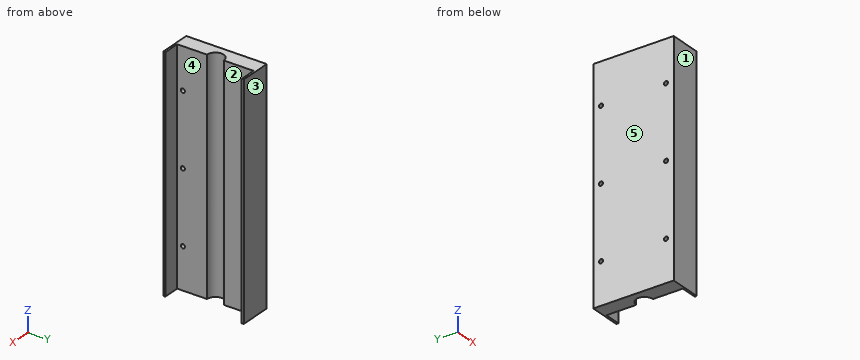
```python
from build123d import *

# Parameters (mm, degrees)
SALIENTE_EXTRUIR1_DEPTH   = 220
CROQUIS5_R                = 2
CORTAR_EXTRUIR5_DEPTH     = 20
CROQUIS7_W                = 220
CROQUIS7_H                = 2
SALIENTE_EXTRUIR2_DEPTH   = 16
SALIENTE_EXTRUIR2_2_DEPTH = 16
CROQUIS7_3_W              = 220
CROQUIS7_3_H              = 2
SALIENTE_EXTRUIR3_DEPTH   = 15


with BuildPart() as part:
    # Croquis1 → Saliente-Extruir1 (new body)
    with BuildSketch(Plane.XY):
        with BuildLine():
            Line((0, 37), (0, 8.15))
            ThreePointArc((0, 8.15), (-8.15, 0), (0, -8.15))
            Line((0, -8.15), (0, -37))
            Line((0, -37), (-15, -37))
            Line((-15, -37), (-15, 37))
            Line((-15, 37), (0, 37))
        make_face()
    extrude(amount=SALIENTE_EXTRUIR1_DEPTH)

    # Croquis5 → Cortar-Extruir5 (cut)
    with BuildSketch(Plane.ZY.offset(15)):
        with Locations((110, -31.5)):
            Circle(CROQUIS5_R)
        with Locations((110, 31.5)):
            Circle(CROQUIS5_R)
        with Locations((40, 31.5)):
            Circle(CROQUIS5_R)
        with Locations((40, -31.5)):
            Circle(CROQUIS5_R)
        with Locations((180, 31.5)):
            Circle(CROQUIS5_R)
        with Locations((180, -31.5)):
            Circle(CROQUIS5_R)
    extrude(amount=-CORTAR_EXTRUIR5_DEPTH, mode=Mode.SUBTRACT)



with BuildPart() as body_2:
    # Croquis7 → Saliente-Extruir2 (new body)
    with BuildSketch(Plane(origin=(0, 0, 0), x_dir=(0, 0, -1), z_dir=(1, 0, 0))):
        with Locations((-110, -38)):
            Rectangle(CROQUIS7_W, CROQUIS7_H)
    extrude(amount=SALIENTE_EXTRUIR2_DEPTH)


with BuildPart() as body_3:
    # Croquis7 → Saliente-Extruir2 2 (new body)
    with BuildSketch(Plane(origin=(0, 0, 0), x_dir=(0, 0, -1), z_dir=(1, 0, 0))):
        with Locations((-110, 38)):
            Rectangle(CROQUIS7_W, CROQUIS7_H)
    extrude(amount=SALIENTE_EXTRUIR2_2_DEPTH)


with BuildPart() as part_1:
    add(part.part)

    add(body_2.part)  # Saliente-Extruir3 merges body 2

    add(body_3.part)  # Saliente-Extruir3 merges body 3
    # Croquis7_3 → Saliente-Extruir3 (add)
    with BuildSketch(Plane(origin=(0, 0, 0), x_dir=(0, 0, -1), z_dir=(1, 0, 0))):
        with Locations((-110, -38)):
            Rectangle(CROQUIS7_3_W, CROQUIS7_3_H)
        with Locations((-110, 38)):
            Rectangle(CROQUIS7_3_W, CROQUIS7_3_H)
    extrude(amount=-SALIENTE_EXTRUIR3_DEPTH)


solid = part_1.part
```
Check sheet for the modelled part. Datum: model origin and axes. Units: mm. Face numbers are marked on the shaded views. A direction names the side the tool comes from. Round coordinates to 2 decimals unless told otherwise and drop trailing zeros. Order: outer loops, then holes, each group sorted by start corner. A loop starts at its lowest first (then second) coordinate and runs counter-clockwise, first axis right, second up. Notation, with made-up numbers: (84.25, 19) -> (100.25, 19) arc R19 cw to (100.25, 53) -> close; hole circle Ø2 at (81, 79.5). An arc over 180 degrees is marked (long way). One line per item, written item: value. Start each with the question number.
Q1. Cross-section at A-A (x = 9.5). Record the boundary of the cut face in (y, z), and give its area (3 significant figures).
Q2. Cross-section at D-D (y = -26). Record the boundary of the cut face in (x, z).
Q3. Cross-section at B-B (z = 180). Record the boundary of the cut face in (x, y), and give its area (3 significant figures).
Q4. Cross-section at C-C (x = -2). Record the boundary of the cut face in (y, z), and give its area (3 significant figures).
Q5. Thickness scan on line 1 (Y direction, x = -10.25, z = 40); line 2 (Z direction, x = -10, y = -31); line 3 (Y direction, x = 15, z = 51). Record the ranges inside material, lowest first.
Q6. Set-up check for the marked faces 4 and 5: record each of +Z, -Z, +X, -X, +Y, -Y from which the full face is reachable in a straight line by a thin tool's end or side.
Q7. Mould release check, pull along Y, two halves, no side actions. Record for the marked faces 1, 2 and 3: pulls with the +Y half, pulls with the -Y half, needs draft (parallel to the pull), parting line crosses it, or undercut.
Q8. Gauge pin test, flat end, axial feed: pin 1 Ø8.5 at (y, z) = (-18.5, 114.5) entering from +X. Record the tip position at first contact, or that the pin passes through.
Completed:
1. outline: (-39, 0) -> (-37, 0) -> (-37, 220) -> (-39, 220) -> close; (37, 0) -> (39, 0) -> (39, 220) -> (37, 220) -> close
1. area: 880 mm²
2. outline: (-15, 0) -> (0, 0) -> (0, 220) -> (-15, 220) -> close
3. outline: (-15, -39) -> (16, -39) -> (16, -37) -> (0, -37) -> (0, -33.5) -> (-15, -33.5) -> close; (-15, -29.5) -> (0, -29.5) -> (0, -8.15) arc R8.15 cw to (0, 8.15) -> (0, 29.5) -> (-15, 29.5) -> close; (-15, 33.5) -> (0, 33.5) -> (0, 37) -> (16, 37) -> (16, 39) -> (-15, 39) -> close
3. area: 1,010 mm²
4. outline: (-39, 0) -> (-7.9, 0) -> (-7.9, 220) -> (-39, 220) -> close; (7.9, 0) -> (39, 0) -> (39, 220) -> (7.9, 220) -> close; hole circle Ø4 at (-31.5, 40); hole circle Ø4 at (-31.5, 110); hole circle Ø4 at (-31.5, 180); hole circle Ø4 at (31.5, 40); hole circle Ø4 at (31.5, 110); hole circle Ø4 at (31.5, 180)
4. area: 13,600 mm²
5. line 1: y = -39 to -33.5, -29.5 to 29.5, 33.5 to 39
5. line 2: z = 0 to 38.06, 41.94 to 108.06, 111.94 to 178.06, 181.94 to 220
5. line 3: y = -39 to -37, 37 to 39
6. face 4: +Z, -Z, +X
6. face 5: +Z, -Z, -X, +Y, -Y
7. face 1: pulls with the -Y half
7. face 2: undercut
7. face 3: pulls with the +Y half
8. pin 1: stops at x = 0
